Autodesk Inventor part; units mm, degrees
ref_plane "YZ 平面" through (0, 0, 0) normal (1, 0, 0) x (0, 1, 0)
ref_plane "XZ 平面" through (0, 0, 0) normal (0, 1, 0) x (-1, 0, 0)
ref_plane "XY 平面" through (0, 0, 0) normal (0, 0, 1) x (1, 0, 0)
sketch "草圖1" plane through (0, 0, 0) normal (0, 0, 1) x (1, 0, 0)
  line L0 (-8, -63.5) -> (8, -63.5)
  line L1 (8, -63.5) -> (8, 63.5)
  line L2 (8, 63.5) -> (-8, 63.5)
  line L3 (-8, 63.5) -> (-8, -63.5)
  line L4 (-8, -63.5) -> (8, 63.5) construction
  line L5 (8, -63.5) -> (-8, 63.5) construction
  point P0 (0, 0)
  dimension "d0" = 16
  dimension "d1" = 127
extrude "擠出1" add sketch "草圖1" along normal blind 6
sketch "草圖2" plane through (0, 0, 6) normal (0, 0, 1) x (1, 0, 0)
  line L0 (-5.5, -61) -> (5.5, -61)
  line L1 (5.5, -61) -> (5.5, 49)
  line L2 (5.5, 49) -> (-5.5, 49)
  line L3 (-5.5, 49) -> (-5.5, -61)
  line L4 (-5.5, -61) -> (5.5, 49) construction
  line L5 (5.5, -61) -> (-5.5, 49) construction
  line L6 (-8, -63.5) -> (8, -63.5)
  line L7 (8, -63.5) -> (8, 63.5)
  point P0 (0, 0)
  point P1 (0, -6)
  dimension "d4" = 11
  dimension "d5" = 110
  dimension "d6" = 2.5
  dimension "d7" = 2.5
extrude "擠出2" cut sketch "草圖2" against normal blind 3
sketch "草圖3" plane through (0, 0, 3) normal (0, 0, 1) x (1, 0, 0)
  line L0 (-5.5, 49) -> (5.5, 49)
  line L1 (5.5, 49) -> (5.5, 45)
  line L2 (5.5, 45) -> (-5.5, 45)
  line L3 (-5.5, 45) -> (-5.5, 49)
  line L4 (-5.5, 49) -> (5.5, 45) construction
  line L5 (5.5, 49) -> (-5.5, 45) construction
  line L6 (-5.5, 49) -> (5.5, 49)
  line L7 (-5.5, -61) -> (-5.5, 49)
  point P0 (0, 0)
  point P1 (0, 47)
  dimension "d10" = 11
  dimension "d11" = 4
  dimension "d12" = 0
  dimension "d13" = 0
extrude "擠出3" cut sketch "草圖3" against normal blind 3
sketch "草圖4" plane through (0, 0, 6) normal (0, 0, 1) x (1, 0, 0)
  circle A0 centre (0, 56.5) radius 1.5
  line L0 (8, 63.5) -> (-8, 63.5)
  line L1 (-8, 63.5) -> (-8, -63.5)
  point P0 (0, 0)
  dimension "d16" = 7
  dimension "d17" = 8
  dimension "d18" = 3
extrude "擠出4" cut sketch "草圖4" against normal blind 6
chamfer "倒角1" distance 1 angle 45 16 edges at (-5.5, -6, 6) (-8, 0, 6) (8, 0, 6) (5.5, -6, 6) (0, 49, 6) (0, -61, 6) (0, -63.5, 6) (0, 63.5, 6) (8, 63.5, 3) (-8, 63.5, 3) (8, -63.5, 3) (-8, -63.5, 3) (-8, 0, 0) (0, -63.5, 0) (8, 0, 0) (0, 63.5, 0)
sketch "草圖5" plane through (0, 0, 0) normal (0, 0, -1) x (-1, 0, 0)
  circle A0 centre (0, 56.5) radius 3
  line L0 (7, 63.5) -> (-7, 63.5)
  line L1 (8, -62.5) -> (8, 62.5)
  point P0 (0, 0)
  dimension "d24" = 6
  dimension "d25" = 7
  dimension "d26" = 8
extrude "擠出5" cut sketch "草圖5" against normal blind 2
chamfer "倒角2" distance 1 angle 45 2 edges at (0, 45, 0) (0, 49, 0)
chamfer "倒角3" distance 1 angle 45 1 edges at (-5.5, 44.5, 0)
chamfer "倒角4" distance 1 angle 45 1 edges at (5.5, 44.5, 0)
properties part number "風力"
Could you check a few things on this model? Use its own coordinates, in mm. A direction names the side the tool comes from. Give positions to 0.01 mm unless a question says otherwise; leave off trailing zeros. Order: outer loops, then holes, each group sorted by start corner. A loop starts at its lowest first (then second) coordinate and runs counter-clockwise, first axis right, second up. Notation, with made-up numbers: (-35, 53) - (-31, 53) arc R24 ccw to (-31, 76) - close; hole circle Ø7 at (45.5, 47.5). An arc over 180 degrees is marked (long way). One line per item, written item: value. Start each with the question number.
1. Imagine slicing it at B-B on y = -1. List the corners of the cut face in (x, z) for me, plus the area to 3 significant figures.
2. Thinking about a two-plate mould opening in Y: for faces 1 (the face through (-8, 1, 3)), 2 (the face through (0, 63.5, 3)), 3 (the face through (-5.5, -7, 4)), which applies, +Y half, -Y half, draft (parallel to the pull), parting line (faces both ways), or undercut?
3. For faces 4 (the face through (0.391, 59.474, 0.986)), 5 (the face through (5.5, -5, 4)), 6 (the face through (0, 45, 2)), 7 (the face through (8, -1, 3)), 8 (the face through (0, -63.5, 3)), which set-ups out of +Z, -Z, +X, -X, +Y, -Y let a thin tool reach every point of the face, with its end or its side?
4. For P1, Ø2.5, axis at x = 0, y = 56.5, coming from the -Z side; P2, Ø5, axis at x = 3.5, y = -6.5, coming from the +Z side; P3, Ø3.5, axis at x = -1.5, y = -22.5, coming from the +Z side; P4, Ø3, axis at x = 1, y = 57.5, coming from the -Z side, each with a flat end and sliding along its axis, tell me the tip position at first contact or that it passes through.
5. Imagine slicing it at C-C on y = 56.5. List the corners of the cut face in (x, z) for me.
6. If I drill on probe 1 along Y at (x, z) = (0, 3.35); probe 2 along Y at (x, z) = (-0.25, 1.6); probe 3 along Y at (x, z) = (-4, 2.9), over which ranges is the centre line in solid material (lowest first)?
7. Imagine slicing it at A-A on x = 0. List the corners of the cut face in (y, z) for me.
Values:
1. outline: (-8, 1) - (-7, 0) - (7, 0) - (8, 1) - (8, 5) - (7, 6) - (6.5, 6) - (5.5, 5) - (5.5, 3) - (-5.5, 3) - (-5.5, 5) - (-6.5, 6) - (-7, 6) - (-8, 5) - close
1. area: 60.0 mm²
2. face 1: draft
2. face 2: +Y half
2. face 3: undercut
3. face 4: -Z
3. face 5: +Z
3. face 6: +Z, -Z
3. face 7: +Z, -Z, +X, +Y, -Y
3. face 8: +Z, -Z, +X, -X, -Y
4. P1: through
4. P2: z = 5.5
4. P3: z = 3
4. P4: z = 2
5. outline: (-8, 1) - (-7, 0) - (-3, 0) - (-3, 2) - (-1.5, 2) - (-1.5, 6) - (-7, 6) - (-8, 5) - close; (1.5, 2) - (3, 2) - (3, 0) - (7, 0) - (8, 1) - (8, 5) - (7, 6) - (1.5, 6) - close
6. probe 1: -63.5 to -61, 49 to 55, 58 to 63.5
6. probe 2: -63.5 to 45, 49 to 53.51, 59.49 to 63.5
6. probe 3: -63.5 to 45, 49 to 63.5
7. outline: (-63.5, 1) - (-62.5, 0) - (44, 0) - (45, 1) - (45, 3) - (-61, 3) - (-61, 5) - (-62, 6) - (-62.5, 6) - (-63.5, 5) - close; (49, 1) - (50, 0) - (53.5, 0) - (53.5, 2) - (55, 2) - (55, 6) - (50, 6) - (49, 5) - close; (58, 2) - (59.5, 2) - (59.5, 0) - (62.5, 0) - (63.5, 1) - (63.5, 5) - (62.5, 6) - (58, 6) - close
